Can you work these out from the model? Positions are in its coordinate system, mm. Face numbers are marked on the shaded views. A direction names the side the tool comes from. Round coordinates to 2 decimals unless told otherwise and drop trailing zeros. Write each loop counter-clockwise with the first axis right and the second up, starting at its lowest first coordinate (ties: lowest second). Pieces come first, ordered by that corner, then holes. Notation, with made-up numbers: M 14.5,20 L 26.5,20 A8 ccw 26.5,27 Z; hole C -31,35 d3. An arc over 180 degrees is marked long. Answer as a JSON object with one key per item and string values. Group by question number.
1) Suppose I cut it at B-B, the plane x = 0. Write out the boundary of the cut face in (y, z).
2) I'm going to push flat-ended pins straight in: pin 1 Ø1.5 at (x, y) = (-15.5, -3.5) entering from -Z; pin 2 Ø4 at (x, z) = (-14.5, 1) entering from +Y; pin 3 Ø5 at (x, y) = (-18, -8.5) entering from +Z. Where does each tip first touch, or does it pass through?
3) Suppose I cut it at D-D, the plane y = -4. Write out the boundary of the cut face in (x, z).
4) Suppose I cut it at A-A, the plane z = 0. Write out the boundary of the cut face in (x, y), and give its area (3 significant figures).
5) Suppose I cut it at C-C, the plane y = -8.75. Write out the boundary of the cut face in (x, z), and give its area (3 significant figures).
6) On a 3-axis mill with a long thin cutter (end or side, diameter ignored), from which of +Z, -Z, +X, -X, +Y, -Y can I reach the whole of each face in a straight line? I mean the marked faces 4 and 5. Say none if no direction works.
7) Please list where these lines run through material, in increasing order: L1, parallel to Z at x = 0, y = -2.25; L2, parallel to Z at x = 0, y = -9; L3, parallel to Y at x = 3, z = 15. Write a range as [from, to].
8) If we mould it in two halves opening along Z, with no side actions, what happens to the marked faces 1, 2 and 3? For each: +Z half, -Z half, draft (parallel to the pull), parting line (faces both ways), or undercut.
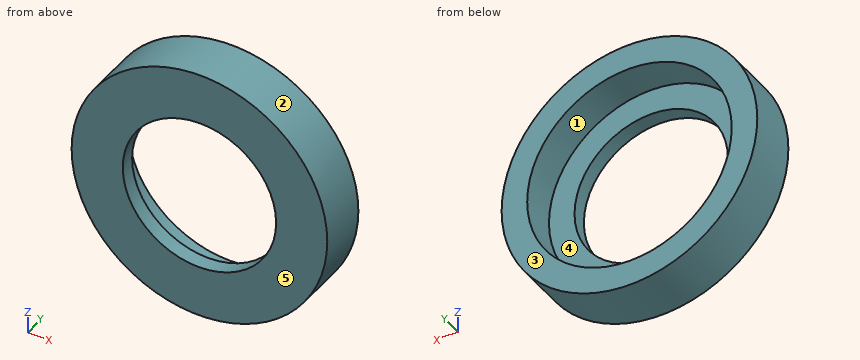
Autodesk Inventor part; units mm, degrees
ref_plane "YZ Plane" through (0, 0, 0) normal (1, 0, 0) x (0, 1, 0)
ref_plane "XZ Plane" through (0, 0, 0) normal (0, 1, 0) x (-1, 0, 0)
ref_plane "XY Plane" through (0, 0, 0) normal (0, 0, 1) x (1, 0, 0)
sketch "Sketch1" plane through (0, 0, 0) normal (0, 1, 0) x (-1, 0, 0)
  circle A0 centre (0, 0) radius 25
  dimension "d0" = 50
extrude "Extrusion1" add sketch "Sketch1" against normal blind 10
sketch "Sketch3" plane through (0, 0, 0) normal (0, 1, 0) x (-1, 0, 0)
  circle A0 centre (0, 0) radius 15
  dimension "d3" = 30
extrude "Extrusion2" cut sketch "Sketch3" against normal blind 10
sketch "Sketch4" plane through (0, 0, 0) normal (0, 1, 0) x (-1, 0, 0)
  circle A0 centre (0, 0) radius 20
  dimension "d6" = 40
extrude "Extrusion3" cut sketch "Sketch4" against normal blind 7
properties part number "Седло для сальника"
Results:
{
 "1": {"outline": "M -10,-25 L 0,-25 L 0,-20 L -7,-20 L -7,-15 L -10,-15 Z; M -10,15 L -7,15 L -7,20 L 0,20 L 0,25 L -10,25 Z"},
 "2": {"pin 1": "z = -20.19", "pin 2": "y = -7", "pin 3": "z = 19.62"},
 "3": {"outline": "C 0,0 d50; hole C 0,0 d40"},
 "4": {"outline": "M -25,-10 L -15,-10 L -15,-7 L -20,-7 L -20,0 L -25,0 Z; M 15,-10 L 25,-10 L 25,0 L 20,0 L 20,-7 L 15,-7 Z", "area": "130 mm^2"},
 "5": {"outline": "C 0,0 d50; hole C 0,0 d30", "area": "1,260 mm^2"},
 "6": {"face 4": "+Y", "face 5": "+Z, -Z, +X, -X, -Y"},
 "7": {"L1": "[-25, -20], [20, 25]", "L2": "[-25, -15], [15, 25]", "L3": "[-10, -7]"},
 "8": {"face 1": "undercut", "face 2": "parting line", "face 3": "draft"}
}
